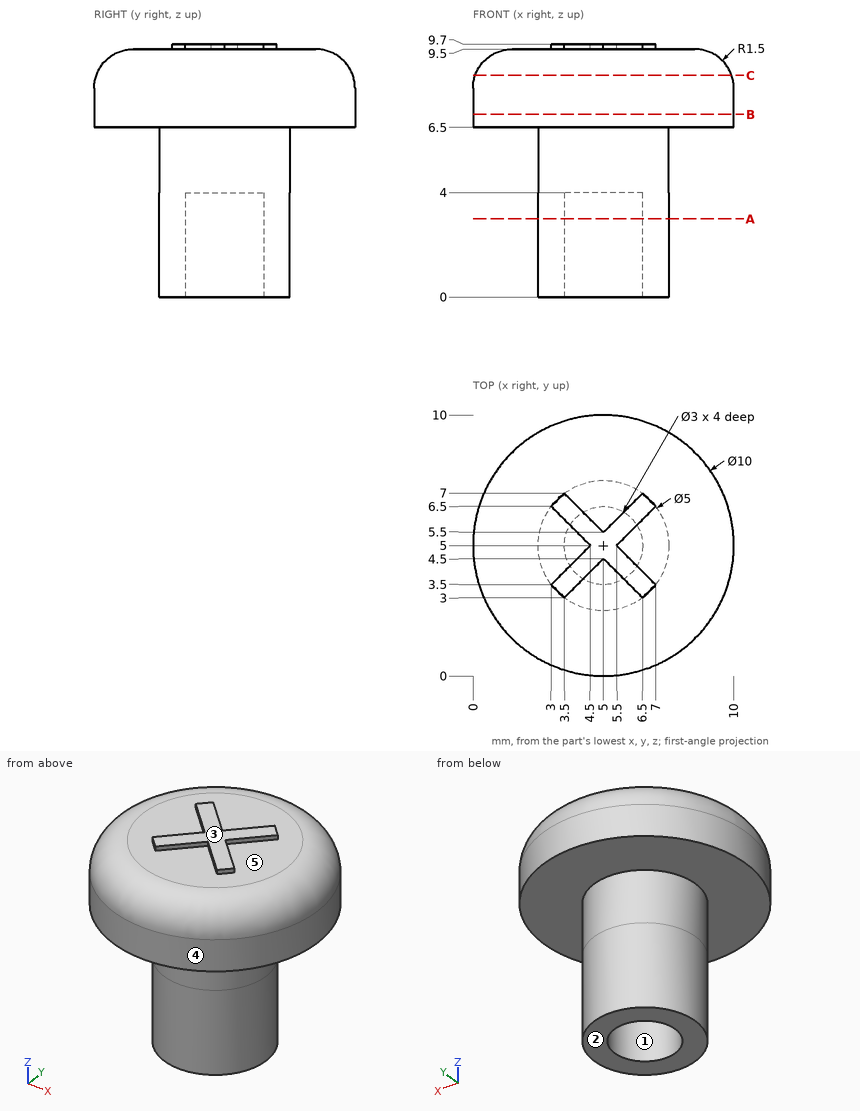
Geometry: see drawing. Coordinates: mm, zero at the bounding-box minimum. A direction names the side the tool comes from. Round coordinates to 2 decimals unless told otherwise and drop trailing zeros. Write each loop counter-clockwise with the first axis right and the second up, starting at its lowest first coordinate (ties: lowest second). Pieces come first, ordered by that corner, then holes.
Item 1: Material intervals for L1, parallel to X at y = 5, z = 2.05; L2, parallel to Z at x = 6, y = 4, sorted ascending.
Item 2: Section query A-A (z = 3). Return loops of the section in (x, y).
Item 3: Set-up query: the marked faces 1 and 2. Return all of +Z, -Z, +X, -X, +Y, -Y with unobstructed straight access to the full face (end or side cutting, diameter ignored); none if empty.
Item 4: Mould query, pull axis Y, two halves, no side actions, for the marked faces 3, 4 and 5. Classes: +Y half, -Y half, draft (parallel to the pull), parting line (faces both ways), or undercut.
Item 5: Section query C-C (z = 8.5). Return loops of the section in (x, y).
Item 6: Pin query (flat end, axial travel): P1, Ø0.9, axis at x = 4.5, y = 5, coming from the -Z side; P2, Ø1, axis at x = 9, z = 3, coming from the -Y side; P3, Ø4, axis at x = 3, z = 1, coming from the -Y side. Return the tip coordinate at first contact, or that it passes through.
Item 7: Section query B-B (z = 7). Return loops of the section in (x, y), plus the area to 3 significant figures.
Completed:
1. L1: x = 2.5 to 3.5, 6.5 to 7.5
1. L2: z = 4 to 9.7
2. outline: circle Ø5 at (5, 5); hole circle Ø3 at (5, 5)
3. face 1: -Z
3. face 2: -Z, +X, -X, +Y, -Y
4. face 3: draft
4. face 4: parting line
4. face 5: undercut
5. outline: circle Ø9.83 at (5, 5)
6. P1: stops at z = 4
6. P2: passes through
6. P3: stops at y = 2.5
7. outline: circle Ø10 at (5, 5)
7. area: 78.5 mm2
